The model under review builds one solid part; all positions refer to its coordinate system, in mm. A direction names the side the tool comes from. Coordinates: 2 decimals unless noted, no trailing zeros. Order: outer loops, then holes, each group sorted by start corner. A loop starts at its lowest first (then second) coordinate and runs counter-clockwise, first axis right, second up.
```python
from build123d import *

# Parameters (mm, degrees)
SKETCH1_R           = 5
SKETCH1_R_2         = 2.5
BOSS_EXTRUDE1_DEPTH = 200
SKETCH2_W           = 20
SKETCH2_H           = 2
CUT_EXTRUDE1_DEPTH  = 40
CUT_EXTRUDE2_START  = -70
SKETCH4_W           = 20
SKETCH4_H           = 2
CUT_EXTRUDE2_DEPTH  = 271.124960962


with BuildPart() as part:
    # Sketch1 → Boss-Extrude1 (new body)
    # profile 1 of 2: a face of its own
    with BuildSketch(Plane.XY):
        Circle(SKETCH1_R)
        Circle(SKETCH1_R_2, mode=Mode.SUBTRACT)
    # profile 2 of 2: a face of its own
    with BuildSketch(Plane.XY):
        Circle(SKETCH1_R_2)
    extrude(amount=-BOSS_EXTRUDE1_DEPTH)

    # Sketch2 → Cut-Extrude1 (cut)
    with BuildSketch(Plane.XY):
        with Locations((0, 5)):
            Rectangle(SKETCH2_W, SKETCH2_H)
    extrude(amount=-CUT_EXTRUDE1_DEPTH, mode=Mode.SUBTRACT)

    # Sketch4 → Cut-Extrude2 (cut, through all)
    with BuildSketch(Plane(origin=(0, 0, -200), x_dir=(-1, 0, 0), z_dir=(0, 0, -1)).offset(CUT_EXTRUDE2_START)):
        with Locations((0, 5)):
            Rectangle(SKETCH4_W, SKETCH4_H)
    extrude(amount=CUT_EXTRUDE2_DEPTH, mode=Mode.SUBTRACT)


solid = part.part
```
(1) We need section A-A, the plane x = 0. Write out the cut boundary in (y, z).
A:
outline: (-5, -200) - (4, -200) - (4, -130) - (5, -130) - (5, -40) - (4, -40) - (4, 0) - (-5, 0) - close
(2) Wall thickness on probe 1 along X at (y, z) = (-0.25, -74.5); probe 2 along Z at (x, y) = (-2.25, 4.25); probe 3 along X at (y, z) = (-0.75, -136.5): over which ranges is each line inside the solid? List them lowest first.
A:
probe 1: x = -4.99 to 4.99
probe 2: z = -130 to -40
probe 3: x = -4.94 to 4.94
(3) We need section C-C, the plane y = -3.25. Write out the cut boundary in (x, z).
A:
outline: (-3.8, -200) - (3.8, -200) - (3.8, 0) - (-3.8, 0) - close
(4) For pin 1 Ø1.8 at (x, z) = (0.5, -180) entering from +Y; pin 2 Ø1 at (y, z) = (3, -76) entering from -X, all flat-tipped, find the tip position at first contact; note any pin that passes through.
A:
pin 1: stops at y = 4
pin 2: stops at x = -4.33
(5) Machinability: for faces 1 (the face through (0, 0, 0)), 2 (the face through (0, 4, -20)), 3 (the face through (0, 4, -165)), which of the approach directions +Z, -Z, +X, -X, +Y, -Y give a long, thin tool a straight path to every point of the face, cutting with its end or side? Answer none if there is none.
A:
face 1: +Z, +X, -X, +Y, -Y
face 2: +Z, +X, -X, +Y
face 3: -Z, +X, -X, +Y
(6) We need section B-B, the plane z = -113. Write out the cut boundary in (x, y), and give its area (3 significant figures).
A:
outline: circle Ø10 at (0, 0)
area: 78.5 mm2
